Autodesk Inventor part; units mm, degrees
ref_plane "YZ Plane" through (0, 0, 0) normal (1, 0, 0) x (0, 1, 0)
ref_plane "XZ Plane" through (0, 0, 0) normal (0, 1, 0) x (-1, 0, 0)
ref_plane "XY Plane" through (0, 0, 0) normal (0, 0, 1) x (1, 0, 0)
sketch "Sketch1" plane through (0, 0, 0) normal (0, 1, 0) x (-1, 0, 0)
  line L0 (25, 25) -> (-25, 25)
  line L1 (-25, 25) -> (-25, -25)
  line L2 (-25, -25) -> (25, -25)
  line L3 (25, -25) -> (25, 25)
  point P0 (0, 0)
  dimension "d0" = 50
  dimension "d1" = 50
  dimension "d2" = 25
  dimension "d3" = 25
extrude "Extrusion1" add sketch "Sketch1" along normal blind 5
sketch "Sketch2" plane through (0, 0, 0) normal (0, -1, 0) x (1, 0, 0)
  circle A0 centre (0, 0) radius 8
  dimension "d6" = 16
extrude "Extrusion2" add sketch "Sketch2" along normal blind 10
sketch "Sketch3" plane through (0, 5, 0) normal (0, 1, 0) x (1, 0, 0)
  line L0 (0, -3) -> (0, -3)
  line L1 (3, 0) -> (3, 0)
  line L2 (0, 3) -> (0, 3)
  line L3 (-3, 0) -> (-3, 0)
  arc A0 (-3, 0) -> (0, -3) centre (0, 0) ccw
  arc A1 (0, 3) -> (-3, 0) centre (0, 0) ccw
  arc A2 (3, 0) -> (0, 3) centre (0, 0) ccw
  arc A3 (0, -3) -> (3, 0) centre (0, 0) ccw
  point P0 (0, 0)
  dimension "d9" = 6
  dimension "d10" = 6
  dimension "d11" = 3
  dimension "d12" = 3
  dimension "d19" = 3
extrude "Extrusion3" cut sketch "Sketch3" against normal blind 6
sketch "Sketch4" plane through (0, 5, 0) normal (0, 1, 0) x (1, 0, 0)
  line L0 (-5, -5) -> (-5, 5)
  line L1 (-25, 25) -> (-25, -25)
  circle A0 centre (-15, 0) radius 2.5
  line L2 (5, -5) -> (-5, -5)
  line L3 (-5, 5) -> (5, 5)
  circle A1 centre (15, 0) radius 2.5
  line L4 (25, -25) -> (25, 25)
  point P0 (0, 0)
  dimension "d15" = 5
  dimension "d20" = 10
  dimension "d21" = 10
extrude "Extrusion4" cut sketch "Sketch4" against normal blind 3
fillet "Fillet1" radius 5 4 edges at (25, 2.5, 25) (25, 2.5, -25) (-25, 2.5, -25) (-25, 2.5, 25)
sketch "Sketch5" plane through (0, 0, 0) normal (1, 0, 0) x (0, 1, 0)
  line L0 (0, 8) -> (-10, 8)
  line L1 (0, 8) -> (0, 8.25)
  line L2 (0, 20) -> (0, -20)
  line L3 (-10, 8) -> (-10, -8)
  line L4 (0, 8.25) -> (-10, 8)
  line L5 (-10, 8) -> (0, 8)
  line L6 (-10, 0) -> (0, 0)
  dimension "d23" = 0.25
revolve "Revolution1" add sketch "Sketch5" angle 360 about axis through (0, -10, 0) along (0, 1, 0) contours L0 L4 L1
properties part number "Base2"
Verification items for the finished model (mm, model axes). A direction names the side the tool comes from. Coordinates: 2 decimals unless noted, no trailing zeros. Write each loop counter-clockwise with the first axis right and the second up, starting at its lowest first coordinate (ties: lowest second). Pieces come first, ordered by that corner, then holes. Notation, with made-up numbers: (63, 17) - (74, 17) arc R5 cw to (74, 23) - close; hole circle Ø3 at (18, -2). An arc over 180 degrees is marked (long way). One line per question, with ' | ' between items. Start each with the question number.
1. Gauge pin test, flat ends, axial feed: P1, Ø1.5, axis at x = 8.5, z = -6.5, coming from the -Y side; P2, Ø5.5, axis at x = 16, z = 0.5, coming from the +Y side; P3, Ø4, axis at x = -2.5, y = -4, coming from the +Z side; P4, Ø1.5, axis at x = -16, z = -0.5, coming from the +Y side. Record the tip position at first contact, or that the pin passes through.
2. Access from +Z, -Z, +X, -X, +Y, -Y to the whole of each face (thin tool, end or side, straight path). Record for faces 1 (the flat face through (0, -1, 0)), 2 (the flat face through (6, 0, 6)), 3 (the flat face through (25, 2, 0)).
3. Section check C-C (z = 0). Enter the section's corners in (x, y), plus the area to 4 significant figures.
4. Section check D-D (x = 0). Enter the section's corners in (y, z), plus the area to 4 significant figures.
5. Section check A-A (y = 3). Enter the section's corners in (x, z).
6. Section check B-B (x = 15). Enter the section's corners in (y, z), plus the area to 3 significant figures.
7. Draft check along Z on faces 4 (the flat face through (15, 2, 0)), 5 (the cylindrical face through (23, 3, 24)), 6 (the flat face through (0, 2, -25)). Enter one of: released by +Z, released by -Z, zero draft, split by the parting line, or undercut.
8. Material ranges on line 1 along X through (y, z) = (3.9, 0); line 2 along Z through (x, y) = (0, 1.95); line 3 along Z through (x, y) = (15, 4.45), recorded low to high.
Computed values:
1) P1: y = 0 | P2: y = 5 | P3: z = 8.14 | P4: y = 2
2) face 1: +Y | face 2: -Y | face 3: +Z, -Z, +X, +Y, -Y
3) outline: (-25, 0) - (-8.25, 0) - (-8, -10) - (8, -10) - (8.25, 0) - (25, 0) - (25, 5) - (17.5, 5) - (17.5, 2) - (12.5, 2) - (12.5, 5) - (3, 5) - (3, -1) - (-3, -1) - (-3, 5) - (-12.5, 5) - (-12.5, 2) - (-17.5, 2) - (-17.5, 5) - (-25, 5) - close | area: 346.5 mm²
4) outline: (-10, -8) - (0, -8.25) - (0, -25) - (5, -25) - (5, -3) - (-1, -3) - (-1, 3) - (5, 3) - (5, 25) - (0, 25) - (0, 8.25) - (-10, 8) - close | area: 376.5 mm²
5) outline: (-25, -20) arc R5 ccw to (-20, -25) - (20, -25) arc R5 ccw to (25, -20) - (25, 20) arc R5 ccw to (20, 25) - (-20, 25) arc R5 ccw to (-25, 20) - close; hole circle Ø5 at (-15, 0); hole circle Ø6 at (0, 0); hole circle Ø5 at (15, 0)
6) outline: (0, -25) - (5, -25) - (5, -2.5) - (2, -2.5) - (2, 2.5) - (5, 2.5) - (5, 25) - (0, 25) - close | area: 235 mm²
7) face 4: undercut | face 5: released by +Z | face 6: released by -Z
8) line 1: -25 to -17.5, -12.5 to -3, 3 to 12.5, 17.5 to 25 | line 2: -25 to -3, 3 to 25 | line 3: -25 to -2.5, 2.5 to 25
